Check sheet for the modelled part. Datum: model origin and axes. Units: mm. A direction names the side the tool comes from. Give positions to 0.01 mm unless a question says otherwise; leave off trailing zeros. Order: outer loops, then holes, each group sorted by start corner. A loop starts at its lowest first (then second) coordinate and runs counter-clockwise, first axis right, second up. Notation, with made-up numbers: M -12,-12.75 L 13,-12.75 A18 cw 13,-3.75 Z; hole C 11,60 d1. An arc over 180 degrees is marked long. Return JSON: item names as keys, results as strings. Group by question number.
from build123d import *

# Parameters (mm, degrees)
CORTAR_EXTRUIR1_DEPTH = 6.35
CHAFL_N1_SIZE         = 0.9652


with BuildPart() as part:
    # Croquis1 → Revolución1 (revolve)
    with BuildSketch(Plane.XY, mode=Mode.PRIVATE) as revoluci_n1_sk:
        Polygon((0, 41.275), (7.112, 41.275), (7.112, 31.75), (8.636, 31.75), (8.636, 29.3624), (4.826, 29.3624), (4.826, 0), (0, 0), align=None)
    revolve(revoluci_n1_sk.sketch.rotate(Axis((0, 0, 0), (0, 1, 0)), 90), axis=Axis((0, 0, 0), (0, 1, 0)))

    # Croquis2 → Cortar-Extruir1 (cut)
    with BuildSketch(Plane(origin=(0, 41.275, 0), x_dir=(1, 0, 0), z_dir=(0, 1, 0))):
        Polygon((-2.295025055, 3.9751), (-4.59005011, 0), (-2.295025055, -3.9751), (2.295025055, -3.9751), (4.59005011, 0), (2.295025055, 3.9751), align=None)
    extrude(amount=-CORTAR_EXTRUIR1_DEPTH, mode=Mode.SUBTRACT)

    # Chaflán1
    chafl_n1_edges = [part.edges().sort_by_distance(p)[0] for p in [
        (0, 0, 4.826),
        (0, 41.275, 7.112),
    ]]
    chamfer(chafl_n1_edges, length=CHAFL_N1_SIZE)


solid = part.part
1) Depth check by flat-ended pin: P1, Ø5, axis at x = 0, y = 38.5, coming from the -Z side; P2, Ø1.5, axis at x = 5, z = 0.5, coming from the -Y side; P3, Ø1, axis at x = 0, y = 28.5, coming from the -Z side. Enter the tip coordinate at first touch or a pass-through.
2) Release check for a two-part mould opening along Z. For faces 4 (the face through (4, 41.275, -1.5)), 5 (the face through (-8.563, 30.539, 1.124)), 6 (the face through (-3.46, 38.14, 1.96)) record: released by +Z, released by -Z, zero draft, split by the parting line, or undercut.
3) Sectioned sample at A-A on x = 0. Record the boundary of the cut face in (y, z) (3 decimals).
4) Material ranges on line 1 along X through (y, z) = (38, 0); line 2 along Y through (x, z) = (-5.75, 4.5); line 3 along Y through (x, z) = (-1, 5) (3 decimals), recorded low to high.
5) Sectioned sample at B-B on y = 17. Record the boundary of the cut face in (x, z), then the cut area to 3 significant figures.
6) Tool access check on faces 1 (the face through (2.937, 14.965, 3.83)), 2 (the face through (6.943, 35.97, 1.542)), 3 (the face through (0, 0, 0)). Record the directions out of +Z, -Z, +X, -X, +Y, -Y that give a thin tool (end or side, any length) a straight path to the whole face; none if there is none.
Reply:
{
 "1": {"P1": "z = -7.11", "P2": "y = 0.41", "P3": "z = -4.83"},
 "2": {"face 4": "zero draft", "face 5": "split by the parting line", "face 6": "undercut"},
 "3": {"outline": "M 0,-3.861 L 0.965,-4.826 L 29.362,-4.826 L 29.362,-8.636 L 31.75,-8.636 L 31.75,-7.112 L 40.31,-7.112 L 41.275,-6.147 L 41.275,-3.975 L 34.925,-3.975 L 34.925,3.975 L 41.275,3.975 L 41.275,6.147 L 40.31,7.112 L 31.75,7.112 L 31.75,8.636 L 29.362,8.636 L 29.362,4.826 L 0.965,4.826 L 0,3.861 Z"},
 "4": {"line 1": "-7.11 to -4.59, 4.59 to 7.11", "line 2": "29.36 to 31.75", "line 3": "29.362 to 41.275"},
 "5": {"outline": "C 0,0 d9.65", "area": "73.2 mm^2"},
 "6": {"face 1": "-Y", "face 2": "+Y", "face 3": "+Z, -Z, +X, -X, -Y"}
}
